Geometry: final body of the model. Coordinates: model frame, mm. Give positions to 0.01 mm unless a question says otherwise; leave off trailing zeros. Write each loop counter-clockwise with the first axis right and the second up, starting at its lowest first coordinate (ties: lowest second). Pieces come first, ordered by that corner, then holes.
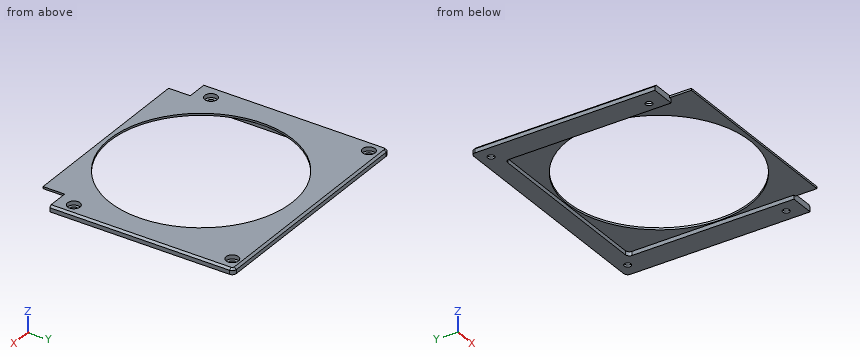
Autodesk Inventor part; units mm, degrees
ref_plane "YZ Plane" through (0, 0, 0) normal (1, 0, 0) x (0, 1, 0)
ref_plane "XZ Plane" through (0, 0, 0) normal (0, 1, 0) x (-1, 0, 0)
ref_plane "XY Plane" through (0, 0, 0) normal (0, 0, 1) x (1, 0, 0)
ref_plane "Work Plane1" through (0, 0, -0.1) normal (0, 0, 1) x (1, 0, 0)
sketch "Sketch1" plane through (0, 0, -0.1) normal (0, 0, 1) x (1, 0, 0)
  circle A0 centre (-100.824, -72) radius 2
  circle A1 centre (2.867, -72) radius 2
  circle A2 centre (-101.9061, 6.8071) radius 2
  circle A3 centre (2.0738, 7.307) radius 2
  spline S0 degree 3 poles (-108.332, 10.6) (-108.332, 10.8554) (-108.2821, 11.108) (-108.0875, 11.5833) (-107.9438, 11.8006) (-107.5783, 12.1734) (-107.3584, 12.3239) (-106.9863, 12.4852) (-106.8508, 12.528) (-106.5731, 12.5855) (-106.4315, 12.6) (-106.2896, 12.6) knots 0 0 0 0 0.240766 0.240766 0.484156 0.484156 0.732838 0.732838 0.866308 0.866308 1 1 1 1
  line L0 (-108.332, 10.6) -> (-108.332, -80)
  line L1 (-96.066, -80) -> (-108.332, -80)
  line L2 (-96.066, -80) -> (-96.066, 1.6)
  arc A4 (-94.066, 3.6) -> (-96.066, 1.6) centre (-94.066, 1.6) ccw
  line L3 (-94.066, 3.6) -> (-5.266, 3.6)
  arc A5 (-3.266, 1.6) -> (-5.266, 3.6) centre (-5.266, 1.6) ccw
  line L4 (-3.266, -80) -> (-3.266, 1.6)
  line L5 (-3.266, -80) -> (9, -80)
  line L6 (9, 10.6) -> (9, -80)
  spline S1 degree 3 poles (6.9576, 12.6) (7.2289, 12.6) (7.4978, 12.5471) (7.9966, 12.3419) (8.2225, 12.1926) (8.5986, 11.8187) (8.7467, 11.5995) (8.9481, 11.1175) (9, 10.8602) (9, 10.6) knots 0 0 0 0 0.255338 0.255338 0.507826 0.507826 0.754805 0.754805 1 1 1 1
  line L7 (-106.2896, 12.6) -> (6.9576, 12.6)
  point P0 (0, 0)
extrude "Extrusion1" add sketch "Sketch1" along normal blind 2 contours A0 | A1 | A2 | A3 | S0 L7 S1 L6 L5 L4 A5 L3 A4 L2 L1 L0
sketch "Sketch2" plane through (0, 0, 1.9) normal (0, 0, 1) x (1, 0, 0)
  line L0 (9, -80) -> (9, 10.6)
  ellipse E0 centre (6.9576, 10.6) end of major axis (9, 10.6) minor radius 2 (9, 10.6) -> (6.9576, 12.6) ccw
  line L1 (6.9576, 12.6) -> (-106.2896, 12.6)
  ellipse E1 centre (-106.2896, 10.6) end of major axis (-104.2473, 10.5998) minor radius 2 (-106.2896, 12.6) -> (-108.332, 10.6) ccw
  line L2 (-108.332, 10.6) -> (-108.332, -80)
  line L3 (8.2, -80) -> (8.2, 10.6)
  line L4 (6.9576, 11.8) -> (-106.2896, 11.8)
  line L5 (-107.532, 10.6) -> (-107.532, -80)
  circle A0 centre (-49.666, -42.9) radius 0.5
  circle A1 centre (-49.666, -42.9) radius 46
  line L6 (8.2, -80) -> (-2.2, -80)
  line L7 (-2.2, -80) -> (-2.2, -90.9)
  line L8 (-2.2, -90.9) -> (-97.166, -90.9)
  line L9 (-97.166, -90.9) -> (-97.166, -80)
  line L10 (-97.166, -80) -> (-107.532, -80)
  line L11 (-2, -97.7) -> (-2, -80.1)
  line L12 (-97.366, -97.7) -> (-97.366, -80.1)
  spline S0 degree 4 poles (8.2, 10.6) (8.1999, 10.8352) (8.1361, 11.0703) (7.879, 11.4945) (7.4469, 11.738) (7.2023, 11.8) (6.9576, 11.8) knots 0 0 0 0 0 0.490114 0.490114 1 1 1 1 1
  spline S1 degree 4 poles (-106.2896, 11.8) (-106.5343, 11.8) (-106.7789, 11.738) (-107.211, 11.4945) (-107.4681, 11.0703) (-107.5319, 10.8352) (-107.532, 10.6) knots 0 0 0 0 0 0.509886 0.509886 1 1 1 1 1
  point P0 (0, 0)
  point P1 (-96.066, -80)
  point P2 (-3.266, -80)
  dimension "d2" = 0.8
  dimension "d3" = 92
  dimension "d6" = 48
  dimension "d25" = 0.2
  dimension "d26" = 0.2
extrude "Extrusion2" add sketch "Sketch2" along normal blind 1 contours L6 L7 L8 L9 L10 L5 S1 L4 S0 L3
sketch "Sketch3" plane through (0, 0, 2.9) normal (0, 0, 1) x (1, 0, 0)
  circle A0 centre (2.0738, 7.307) radius 2 construction
  circle A1 centre (2.867, -72) radius 2 construction
  circle A2 centre (-100.824, -72) radius 2 construction
  circle A3 centre (-101.9061, 6.8071) radius 2 construction
  point P0 (0, 0)
hole "Hole1" at (2.0738, 7.307, 2.9) at (-101.9061, 6.8071, 2.9) at (-100.824, -72, 2.9) at (2.867, -72, 2.9) direction (0, 0, -1) diameter 3.4 end through all counterbore diameter 6.3 counterbore depth 2
sketch "Sketch4" plane through (0, 0, 1.9) normal (0, 0, 1) x (1, 0, 0)
  line L0 (8.2, 10.6) -> (8.2, -80)
  line L1 (8.2, -80) -> (9, -80)
  line L2 (9, -80) -> (9, 10.6)
  ellipse E0 centre (6.9576, 10.6) end of major axis (9, 10.6) minor radius 2 (9, 10.6) -> (6.9576, 12.6) ccw
  line L3 (6.9576, 12.6) -> (-106.2896, 12.6)
  ellipse E1 centre (-106.2896, 10.6) end of major axis (-104.2473, 10.5998) minor radius 2 (-106.2896, 12.6) -> (-108.332, 10.6) ccw
  line L4 (-108.332, 10.6) -> (-108.332, -80)
  line L5 (-108.332, -80) -> (-107.532, -80)
  line L6 (-107.532, -80) -> (-107.532, 10.6)
  ellipse E2 centre (-106.2908, 10.6011) end of major axis (-105.0496, 10.6165) minor radius 1.1989 (-106.2896, 11.8) -> (-107.532, 10.6) ccw
  line L7 (-106.2896, 11.8) -> (6.9576, 11.8)
  ellipse E3 centre (6.9588, 10.6011) end of major axis (8.1999, 10.5856) minor radius 1.1989 (8.2, 10.6) -> (6.9576, 11.8) ccw
  point P0 (0, 0)
extrude "Extrusion3" add sketch "Sketch4" along normal blind 1
chamfer "Chamfer1" distance 1 angle 45 5 edges at (-49.666, 12.6, 2.9) (-107.7338, 12.0142, 2.9) (-108.332, -34.7, 2.9) (8.4018, 12.0142, 2.9) (9, -34.7, 2.9)
properties part number "BP_FanCover"
Q1. Section A-A on y = -42.9. Output: boundary loops of the cut face in (x, z), plus the area to 3 significant figures.
Filled sheet:
outline: (-108.33, -0.1) - (-96.07, -0.1) - (-96.07, 1.9) - (-95.67, 1.9) - (-95.67, 2.9) - (-107.33, 2.9) - (-108.33, 1.9) - close; (-3.67, 1.9) - (-3.27, 1.9) - (-3.27, -0.1) - (9, -0.1) - (9, 1.9) - (8, 2.9) - (-3.67, 2.9) - close
area: 73.4 mm2
Q2. Ray query, line 1 along X through (y, z) = (-72, 0.7); line 2 along X through (y, z) = (-8, 1.7); line 3 along Z through (x, y) = (-94, -1). Return the intervals inside material, ascending.
Filled sheet:
line 1: x = -108.33 to -102.52, -99.12 to -96.07, -3.27 to 1.17, 4.57 to 9
line 2: x = -108.33 to -96.07, -3.27 to 9
line 3: z = 1.9 to 2.9
Q3. Section B-B on x = -78. Output: boundary loops of the cut face in (y, z), plus the area to 3 significant figures.
Filled sheet:
outline: (-90.9, 1.9) - (-79.14, 1.9) - (-79.14, 2.9) - (-90.9, 2.9) - close; (-6.66, 1.9) - (3.6, 1.9) - (3.6, -0.1) - (12.6, -0.1) - (12.6, 1.9) - (11.6, 2.9) - (-6.66, 2.9) - close
area: 48.5 mm2
Q4. Pin query (flat end, axial travel): P1, Ø0.8, axis at y = -86.5, z = 2.5, coming from the -X side; P2, Ø4.5, axis at x = 2.07, y = 7.31, coming from the +Z side; P3, Ø1.6, axis at x = -62.5, z = 1, coming from the -Y side. Return the tip coordinate at first contact, or that it passes through.
Filled sheet:
P1: stops at x = -97.17
P2: stops at z = 0.9
P3: stops at y = 3.6
Q5. Section D-D on x = -54. Output: boundary loops of the cut face in (y, z).
Filled sheet:
outline: (-90.9, 1.9) - (-88.7, 1.9) - (-88.7, 2.9) - (-90.9, 2.9) - close; (2.9, 1.9) - (3.6, 1.9) - (3.6, -0.1) - (12.6, -0.1) - (12.6, 1.9) - (11.6, 2.9) - (2.9, 2.9) - close
Q6. Section C-C on y = -72. Count the separate pieces of the cut face and the enclosed holes in it, plus the area to 3 significant figures.
Filled sheet:
separate pieces: 4
enclosed holes: 0
area: 62.1 mm2
